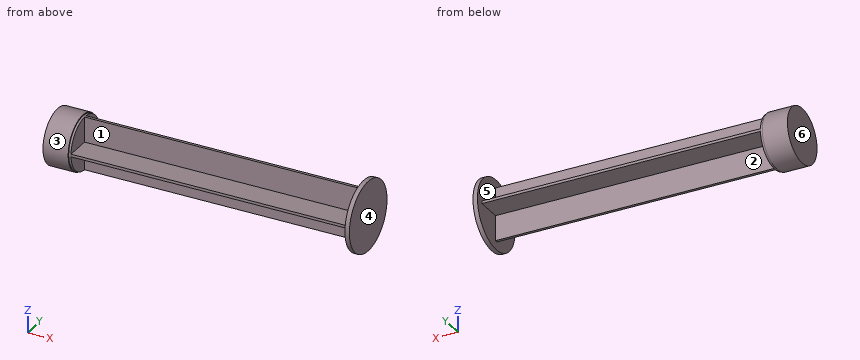
```python
from build123d import *

# Parameters (mm, degrees)
SKETCH1_W           = 1.5
SKETCH1_H           = 14.15
SKETCH1_W_2         = 14.15
SKETCH1_H_2         = 1.5
BOSS_EXTRUDE1_DEPTH = 156.6625
SKETCH2_R           = 19.65
BOSS_EXTRUDE2_DEPTH = 2.5
SKETCH5_W           = 1.3
SKETCH5_H           = 14.9


with BuildPart() as part:
    # Sketch1 → Boss-Extrude1 (new body)
    with BuildSketch(Plane(origin=(0, 0, 0), x_dir=(0, 0, -1), z_dir=(1, 0, 0))):
        with Locations((0.75, -7.075)):
            Rectangle(SKETCH1_W, SKETCH1_H)
        with Locations((8.575, -14.9)):
            Rectangle(SKETCH1_W_2, SKETCH1_H_2)
        with Locations((0.75, -14.9)):
            Rectangle(SKETCH1_W, SKETCH1_H_2)
        with Locations((0.75, -22.725)):
            Rectangle(SKETCH1_W, SKETCH1_H)
        with Locations((-7.075, -14.9)):
            Rectangle(SKETCH1_W_2, SKETCH1_H_2)
    extrude(amount=BOSS_EXTRUDE1_DEPTH)

    # Sketch2 → Boss-Extrude2 (add)
    with BuildSketch(Plane(origin=(156.6625, 0, 0), x_dir=(0, 0, -1), z_dir=(1, 0, 0))):
        with Locations((0.75, -14.9)):
            Circle(SKETCH2_R)
    extrude(amount=BOSS_EXTRUDE2_DEPTH)

    # Sketch5 → Revolve2 (revolve)
    with BuildSketch(Plane(origin=(0, -14.9, 0), x_dir=(1, 0, 0), z_dir=(0, 1, 0)), mode=Mode.PRIVATE) as revolve2_sk:
        Polygon((-15.465, 0.75), (-1.3, 0.75), (-1.3, 15.65), (-1.3, 16.2), (-15.465, 16.2), align=None)
        with Locations((-0.65, 8.2)):
            Rectangle(SKETCH5_W, SKETCH5_H)
    revolve(revolve2_sk.sketch.rotate(Axis((-15.465, -14.9, -0.75), (1, 0, 0)), 180), axis=Axis((-15.465, -14.9, -0.75), (1, 0, 0)))


solid = part.part
```
The model under review builds one solid part; all positions refer to its coordinate system, in mm. Face numbers are marked on the shaded views. A direction names the side the tool comes from. Give positions to 0.01 mm unless a question says otherwise; leave off trailing zeros. Write each loop counter-clockwise with the first axis right and the second up, starting at its lowest first coordinate (ties: lowest second). Pieces come first, ordered by that corner, then holes.
(1) To check wall thickness, follow L1, parallel to X at y = -9.5, z = -7.5 (1 decimal); L2, parallel to Y at x = 119, z = -13; L3, parallel to X at y = -32, z = -3. State the ranges of each line that lie inside material, in increasing order.
(2) For P1, Ø4, axis at x = 104.5, z = 13.5, coming from the -Y side; P2, Ø12, axis at x = 129, y = -21, coming from the +Z side; P3, Ø12, axis at x = 75.5, y = 0.5, coming from the -Z side, all flat-tipped, find the tip position at first contact; note any pin that passes through.
(3) Consider section A-A, the plane x = 105.5. Give the boundary of the cut face in (y, z), and give its area (4 significant figures).
(4) The part is to be moulded in two halves that separate along X. For the marked faces 1, 2, 3 and 4, say which applies: released by +X, released by -X, zero draft, split by the parting line, or undercut.
(5) Tool access review of the marked faces 5 and 6: name each direction out of +Z, -Z, +X, -X, +Y, -Y from which nothing blocks a thin tool from reaching the whole face with its end or side.
(6) Consider section B-B, the plane y = -9. Give the boundary of the cut face in (x, z) (1 decimal), and give its area (3 significant figures).
Returned:
1. L1: x = -15.5 to 0, 156.7 to 159.2
1. L2: y = -15.65 to -14.15
1. L3: x = 156.66 to 159.16
2. P1: stops at y = -15.65
2. P2: stops at z = 14.15
2. P3: stops at z = -1.5
3. outline: (-29.8, -1.5) - (-15.65, -1.5) - (-15.65, -15.65) - (-14.15, -15.65) - (-14.15, -1.5) - (0, -1.5) - (0, 0) - (-14.15, 0) - (-14.15, 14.15) - (-15.65, 14.15) - (-15.65, 0) - (-29.8, 0) - close
3. area: 87.15 mm2
4. face 1: undercut
4. face 2: undercut
4. face 3: zero draft
4. face 4: released by +X
5. face 5: none
5. face 6: +Z, -Z, -X, +Y, -Y
6. outline: (-15.5, -15) - (-1.3, -15) - (-1.3, -14.4) - (0, -14.4) - (0, -1.5) - (156.7, -1.5) - (156.7, -19.5) - (159.2, -19.5) - (159.2, 18) - (156.7, 18) - (156.7, 0) - (0, 0) - (0, 12.9) - (-1.3, 12.9) - (-1.3, 13.5) - (-15.5, 13.5) - close
6. area: 769 mm2
